from build123d import *

# Parameters (mm, degrees)
CUT_EXTRUDE_START   = -2
SKETCH_2_R          = 13.5
CUT_EXTRUDE_3_DEPTH = 2
SKETCH_3_R          = 9.5
CUT_EXTRUDE_4_DEPTH = 0.3
CUT_EXTRUDE_START_2 = -0.3
SKETCH_4_R          = 9.5
CUT_EXTRUDE_5_DEPTH = 0.3


with BuildPart() as part:
    # 草图1 → 旋转1 (revolve)
    with BuildSketch(Plane(origin=(0, 0, 0), x_dir=(0, 0, -1), z_dir=(1, 0, 0)), mode=Mode.PRIVATE) as revolve_1_sk:
        Polygon((0, 8.5), (0, 10.5), (3, 9.5), (3, 13.5), (5, 13.5), (5, 8.5), align=None)
    revolve(revolve_1_sk.sketch.rotate(Axis((0, 0, 0), (0, 0, -1)), 90), axis=Axis((0, 0, 0), (0, 0, -1)))

    # 草图2 → 切除-拉伸3 (cut)
    with BuildSketch(Plane.XY.offset(-3).offset(CUT_EXTRUDE_START)):
        Circle(SKETCH_2_R)
        with BuildLine():
            ThreePointArc((10.499997673, 0.006991234), (10.499999418, 0.003495617), (10.5, 0))
            ThreePointArc((10.5, 0), (10.499999418, -0.003495617), (10.499997673, -0.006991234))
            ThreePointArc((10.499997673, -0.006991234), (11.684968525, -0.591722061), (12.163787272, -1.823305866))
            ThreePointArc((12.163787272, -1.823305866), (11.450680461, -3.269646883), (9.869161474, -3.584641098))
            ThreePointArc((9.869161474, -3.584641098), (9.866772518, -3.591211505), (9.864379188, -3.59778032))
            ThreePointArc((9.864379188, -3.59778032), (10.631190361, -4.270594459), (10.916572605, -5.25))
            ThreePointArc((10.916572605, -5.25), (9.935444894, -6.86715189), (8.047958748, -6.74391281))
            ThreePointArc((8.047958748, -6.74391281), (8.043466653, -6.749269902), (8.038970991, -6.754624002))
            ThreePointArc((8.038970991, -6.754624002), (8.433900995, -7.345998116), (8.572575767, -8.043466653))
            ThreePointArc((8.572575767, -8.043466653), (7.297837999, -9.782293074), (5.256053423, -9.089769107))
            ThreePointArc((5.256053423, -9.089769107), (5.25, -9.09326674), (5.24394425, -9.096760341))
            ThreePointArc((5.24394425, -9.096760341), (5.371363407, -9.472433216), (5.41451737, -9.866772518))
            ThreePointArc((5.41451737, -9.866772518), (3.829501581, -11.674440109), (1.830190483, -10.339265099))
            ThreePointArc((1.830190483, -10.339265099), (1.823305866, -10.340481407), (1.81642044, -10.34169313))
            ThreePointArc((1.81642044, -10.34169313), (1.821583696, -10.420771731), (1.823305866, -10.5))
            ThreePointArc((1.823305866, -10.5), (-0.079228269, -12.321583696), (-1.81642044, -10.34169313))
            ThreePointArc((-1.81642044, -10.34169313), (-1.823305866, -10.340481407), (-1.830190483, -10.339265099))
            ThreePointArc((-1.830190483, -10.339265099), (-4.214818838, -11.580119586), (-5.24394425, -9.096760341))
            ThreePointArc((-5.24394425, -9.096760341), (-5.25, -9.09326674), (-5.256053423, -9.089769107))
            ThreePointArc((-5.256053423, -9.089769107), (-7.921268321, -9.440199979), (-8.038970991, -6.754624002))
            ThreePointArc((-8.038970991, -6.754624002), (-8.043466653, -6.749269902), (-8.047958748, -6.74391281))
            ThreePointArc((-8.047958748, -6.74391281), (-10.672295938, -6.161652933), (-9.864379188, -3.59778032))
            ThreePointArc((-9.864379188, -3.59778032), (-9.866772518, -3.591211505), (-9.869161474, -3.584641098))
            ThreePointArc((-9.869161474, -3.584641098), (-12.136087159, -2.139919606), (-10.499997673, -0.006991234))
            ThreePointArc((-10.499997673, -0.006991234), (-10.5, 0), (-10.499997673, 0.006991234))
            ThreePointArc((-10.499997673, 0.006991234), (-12.136087159, 2.139919606), (-9.869161474, 3.584641098))
            ThreePointArc((-9.869161474, 3.584641098), (-9.866772518, 3.591211505), (-9.864379188, 3.59778032))
            ThreePointArc((-9.864379188, 3.59778032), (-10.672295938, 6.161652933), (-8.047958748, 6.74391281))
            ThreePointArc((-8.047958748, 6.74391281), (-8.043466653, 6.749269902), (-8.038970991, 6.754624002))
            ThreePointArc((-8.038970991, 6.754624002), (-7.921268321, 9.440199979), (-5.256053423, 9.089769107))
            ThreePointArc((-5.256053423, 9.089769107), (-5.25, 9.09326674), (-5.24394425, 9.096760341))
            ThreePointArc((-5.24394425, 9.096760341), (-4.214818838, 11.580119586), (-1.830190483, 10.339265099))
            ThreePointArc((-1.830190483, 10.339265099), (-1.823305866, 10.340481407), (-1.81642044, 10.34169313))
            ThreePointArc((-1.81642044, 10.34169313), (-0.079228269, 12.321583696), (1.823305866, 10.5))
            ThreePointArc((1.823305866, 10.5), (1.821583696, 10.420771731), (1.81642044, 10.34169313))
            ThreePointArc((1.81642044, 10.34169313), (1.823305866, 10.340481407), (1.830190483, 10.339265099))
            ThreePointArc((1.830190483, 10.339265099), (3.829501581, 11.674440109), (5.41451737, 9.866772518))
            ThreePointArc((5.41451737, 9.866772518), (5.371363407, 9.472433216), (5.24394425, 9.096760341))
            ThreePointArc((5.24394425, 9.096760341), (5.25, 9.09326674), (5.256053423, 9.089769107))
            ThreePointArc((5.256053423, 9.089769107), (7.297837999, 9.782293074), (8.572575767, 8.043466653))
            ThreePointArc((8.572575767, 8.043466653), (8.433900995, 7.345998116), (8.038970991, 6.754624002))
            ThreePointArc((8.038970991, 6.754624002), (8.043466653, 6.749269902), (8.047958748, 6.74391281))
            ThreePointArc((8.047958748, 6.74391281), (9.935444894, 6.86715189), (10.916572605, 5.25))
            ThreePointArc((10.916572605, 5.25), (10.631190361, 4.270594459), (9.864379188, 3.59778032))
            ThreePointArc((9.864379188, 3.59778032), (9.866772518, 3.591211505), (9.869161474, 3.584641098))
            ThreePointArc((9.869161474, 3.584641098), (11.450680461, 3.269646883), (12.163787272, 1.823305866))
            ThreePointArc((12.163787272, 1.823305866), (11.684968525, 0.591722061), (10.499997673, 0.006991234))
        make_face(mode=Mode.SUBTRACT)
    extrude(amount=CUT_EXTRUDE_3_DEPTH, mode=Mode.SUBTRACT)

    # 草图3 → 切除-拉伸4 (cut)
    with BuildSketch(Plane.XY):
        Circle(SKETCH_3_R)
    extrude(amount=-CUT_EXTRUDE_4_DEPTH, mode=Mode.SUBTRACT)

    # 草图4 → 切除-拉伸5 (cut)
    with BuildSketch(Plane(origin=(0, 0, -5), x_dir=(-1, 0, 0), z_dir=(0, 0, -1)).offset(CUT_EXTRUDE_START_2)):
        with Locations(Location((0, 0, 0), (0, 0, 180))):
            Circle(SKETCH_4_R)
    extrude(amount=CUT_EXTRUDE_5_DEPTH, mode=Mode.SUBTRACT)


solid = part.part
Here's how the part is built. I have some questions about the finished solid (model axes, mm). A direction names the side the tool comes from. Coordinates: 2 decimals unless noted, no trailing zeros. Order: outer loops, then holes, each group sorted by start corner. A loop starts at its lowest first (then second) coordinate and runs counter-clockwise, first axis right, second up.
Item 1: If we mould it in two halves opening along Z, with no side actions, what happens to faces 3 (the face through (-7.54, 5.78, -4.85)), 4 (the face through (-9, 4, -3)), 5 (the face through (-2.2, -8.4, -0.3))? For each: +Z half, -Z half, draft (parallel to the pull), parting line (faces both ways), or undercut.
Result sheet:
face 3: draft
face 4: undercut
face 5: +Z half
Item 2: For faces 1 (the face through (-2.2, 8.4, -4.7)), 2 (the face through (9, 4, -5)), which set-ups out of +Z, -Z, +X, -X, +Y, -Y let a thin tool reach every point of the face, with its end or its side?
Result sheet:
face 1: -Z
face 2: -Z, +X, -X, +Y, -Y
Item 3: For P1, Ø12, axis at x = -2, y = 3, coming from the +Z side; P2, Ø3, axis at x = -5, z = -2, coming from the +Y side; P3, Ø12, axis at x = 3, y = 1.5, coming from the +Z side; P4, Ø3, axis at x = 3, z = -2, coming from the -Y side, each with a flat end and sliding along its axis, tell me the tip position at first contact or that it passes through.
Result sheet:
P1: stops at z = 0
P2: stops at y = 11.67
P3: stops at z = -0.3
P4: stops at y = -11.69
Item 4: If we section it at B-B on z = -2.3: List the corners of the cut face in (x, y) for me, plus the area to 3 significant figures.
Result sheet:
outline: circle Ø19.47 at (0, 0); hole circle Ø17 at (0, 0)
area: 70.6 mm2
Item 5: I need wall thicknesses on line 1 (Y direction, x = 0, z = -4.9); line 2 (Z direction, x = 0, y = 11.75); line 3 (Z direction, x = -2, y = -8.5). Which ranges of each line are inside material? Lowest first, please.
Result sheet:
line 1: y = -12.32 to -9.5, 9.5 to 12.32
line 2: z = -5 to -3
line 3: z = -4.7 to -0.3
Item 6: If we section it at A-A on x = 0: List the corners of the cut face in (y, z) for me.
Result sheet:
outline: (-12.32, -5) - (-9.5, -5) - (-9.5, -4.7) - (-8.5, -4.7) - (-8.5, -0.3) - (-9.5, -0.3) - (-9.5, 0) - (-10.5, 0) - (-9.5, -3) - (-12.32, -3) - close; (8.5, -4.7) - (9.5, -4.7) - (9.5, -5) - (12.32, -5) - (12.32, -3) - (9.5, -3) - (10.5, 0) - (9.5, 0) - (9.5, -0.3) - (8.5, -0.3) - close
